Autodesk Inventor part; units mm, degrees
ref_plane "YZ Plane" through (0, 0, 0) normal (1, 0, 0) x (0, 1, 0)
ref_plane "XZ Plane" through (0, 0, 0) normal (0, 1, 0) x (-1, 0, 0)
ref_plane "XY Plane" through (0, 0, 0) normal (0, 0, 1) x (1, 0, 0)
sketch "Sketch1" plane through (0, 0, 0) normal (0, 0, 1) x (1, 0, 0)
  line L0 (2, 0) -> (92, 0)
  line L1 (94, 2) -> (94, 42)
  line L2 (92, 44) -> (2, 44)
  line L3 (0, 42) -> (0, 2)
  line L4 (-1, 47) -> (95, 47)
  line L5 (97, 45) -> (97, -1)
  line L6 (95, -3) -> (-1, -3)
  line L7 (-3, -1) -> (-3, 45)
  arc A0 (2, 44) -> (0, 42) centre (2, 42) ccw
  arc A1 (0, 2) -> (2, 0) centre (2, 2) ccw
  arc A2 (92, 0) -> (94, 2) centre (92, 2) ccw
  arc A3 (94, 42) -> (92, 44) centre (92, 42) ccw
  arc A4 (-3, -1) -> (-1, -3) centre (-1, -1) ccw
  arc A5 (-1, 47) -> (-3, 45) centre (-1, 45) ccw
  arc A6 (97, 45) -> (95, 47) centre (95, 45) ccw
  arc A7 (95, -3) -> (97, -1) centre (95, -1) ccw
  point P0 (0, 0)
  point P1 (94, 44)
  point P2 (94, 0)
  point P3 (0, 44)
  point P4 (97, -3)
  point P5 (97, 47)
  point P6 (-3, -3)
  dimension "d0" = 94
  dimension "d1" = 44
  dimension "d2" = 100
  dimension "d3" = 50
  dimension "d4" = 3
  dimension "d5" = 3
  dimension "d6" = 2
  dimension "d9" = 2
extrude "Extrusion1" add sketch "Sketch1" along normal blind 140
sketch "Sketch2" plane through (0, 0, 140) normal (0, 0, 1) x (1, 0, 0)
  line L0 (-3, 45) -> (-3, -1)
  line L1 (97, -1) -> (97, 45)
  line L2 (-3, 32) -> (97, 32)
  line L3 (97, 32) -> (97, 12)
  line L4 (97, 12) -> (-3, 12)
  line L5 (-3, 12) -> (-3, 32)
  line L6 (-1, -3) -> (95, -3)
  line L7 (95, 47) -> (-1, 47)
  point P0 (0, 0)
  point P1 (-3, 12)
  dimension "d10" = 20
  dimension "d11" = 15
  dimension "d12" = 50
extrude "Extrusion2" cut sketch "Sketch2" against normal blind 2
sketch "Sketch3" plane through (97, -1, 0) normal (1, 0, 0) x (0, 0, -1)
  line L0 (-11, 5.5) -> (-36.5, 5.5)
  line L1 (-37.5, 6.5) -> (-37.5, 15.5)
  line L2 (-36.5, 16.5) -> (-11, 16.5)
  line L3 (-10, 15.5) -> (-10, 6.5)
  line L4 (0, -2) -> (-140, -2)
  line L5 (0, 48) -> (-140, 48)
  line L6 (0, 0) -> (0, 46)
  arc A0 (-11, 5.5) -> (-10, 6.5) centre (-11, 6.5) ccw
  arc A1 (-10, 15.5) -> (-11, 16.5) centre (-11, 15.5) ccw
  arc A2 (-37.5, 6.5) -> (-36.5, 5.5) centre (-36.5, 6.5) ccw
  arc A3 (-36.5, 16.5) -> (-37.5, 15.5) centre (-36.5, 15.5) ccw
  circle A4 centre (-7.09, 11) radius 1.5
  circle A5 centre (-40.41, 11) radius 1.5
  line L7 (-23.75, 5.5) -> (-23.75, 19.7829) construction
  point P0 (0, 1)
  point P1 (-37.5, 16.5)
  point P2 (-37.5, 5.5)
  point P3 (-10, 16.5)
  dimension "d15" = 27.5
  dimension "d16" = 11
  dimension "d17" = 50
  dimension "d18" = 31.5
  dimension "d19" = 10
  dimension "d20" = 1
  dimension "d21" = 3
  dimension "d22" = 3
  dimension "d23" = 16.66
  dimension "d24" = 16.66
extrude "Extrusion3" cut sketch "Sketch3" against normal blind 10 contours L0 A2 L1 A3 L2 A1 L3 A0
hole "Hole1" at (97, 10, 7.09) at (97, 10, 40.41) direction (-1, 0, 0) diameter 3.4 depth 8.8 tip angle 118
chamfer "Chamfer1" distance 0.3 angle 45 2 edges at (97, 10, 8.79) (97, 10, 42.11)
sketch "Sketch5" plane through (-1, -3, 0) normal (0, -1, 0) x (1, 0, 0)
  circle A0 centre (45.75, 3.13) radius 1.5
  circle A1 centre (45.75, 97.75) radius 1.5
  line L0 (98, 0) -> (98, 140)
  line L1 (0, 0) -> (96, 0)
  point P0 (1, 0)
  dimension "d49" = 3
  dimension "d50" = 3
  dimension "d51" = 94.62
  dimension "d52" = 52.25
  dimension "d53" = 3.13
hole "Hole3" at (44.75, -3, 3.13) at (44.75, -3, 97.75) direction (0, 1, 0) diameter 2.6416 depth 10.979 tip angle 118
sketch "Sketch6" plane through (0, 0, 0) normal (0, 0, -1) x (-1, 0, 0)
  circle A0 centre (0.8, -0.8) radius 1
  line L0 (1, -3) -> (-95, -3) construction
  line L1 (-47, -3) -> (-47, -11.0585) construction
  line L2 (3, 45) -> (3, -1) construction
  line L3 (3, 22) -> (17.9543, 22) construction
  circle A1 centre (0.8, 44.8) radius 1
  line L4 (-47, 47) -> (-47, 55.0585) construction
  circle A2 centre (-94.8, -0.8) radius 1
  circle A3 centre (-94.8, 44.8) radius 1
  point P0 (0, 0)
  point P1 (-94, 0)
  point P2 (-97, 45)
  point P3 (-97, -1)
  dimension "d61" = 2
  dimension "d62" = 2.2
  dimension "d63" = 2.2
hole "Hole4" at (-0.8, -0.8, 0) at (-0.8, 44.8, 0) at (94.8, 44.8, 0) at (94.8, -0.8, 0) direction (0, 0, 1) diameter 1.567 depth 6.3 tip angle 118
chamfer "Chamfer2" distance 0.2 angle 45 4 edges at (-0.8, -1.5835, 0) (-0.8, 44.0165, 0) (94.8, 44.0165, 0) (94.8, -1.5835, 0)
equation "\"d24\" = d23"
properties part number "obudowa"
Verification items for the finished model (mm, model axes). A direction names the side the tool comes from. Coordinates: 2 decimals unless noted, no trailing zeros. Order: outer loops, then holes, each group sorted by start corner. A loop starts at its lowest first (then second) coordinate and runs counter-clockwise, first axis right, second up. Notation, with made-up numbers: (80.25, 21) - (129.25, 21) arc R21 cw to (129.25, 60) - close; hole circle Ø5 at (53.25, 73). An arc over 180 degrees is marked (long way). Return JSON: item names as keys, results as strings.
(1) Mould release check, pull along X, two halves, no side actions. Record for faces 1 (the flat face through (97, 22, 69)), 2 (the flat face through (0, 22, 69)), 3 (the flat face through (47, 45, 140)), 4 (the flat face through (46, 0, 69)): pulls with the +X half, pulls with the -X half, needs draft (parallel to the pull), parting line crosses it, or undercut.
Filled sheet:
{"face 1": "pulls with the +X half", "face 2": "undercut", "face 3": "needs draft", "face 4": "undercut"}
(2) Section check D-D, the plane y = 17. Record the cut outline in (x, z).
Filled sheet:
{"outline": "(-3, 0) - (0, 0) - (0, 138) - (-3, 138) - close; (94, 0) - (97, 0) - (97, 138) - (94, 138) - close"}
(3) Thickness scan on line 1 along Z through (x, y) = (95.15, 10); line 2 along X through (y, z) = (17.5, 102); line 3 along Y through (x, z) = (22.5, 71.5). Record the ranges inside material, lowest first.
Filled sheet:
{"line 1": "z = 0 to 5.39, 8.79 to 10, 37.5 to 38.71, 42.11 to 140", "line 2": "x = -3 to 0, 94 to 97", "line 3": "y = -3 to 0, 44 to 47"}
(4) Section check A-A, the plane x = 86. Record the cut outline in (y, z), and give its area (3 significant figures).
Filled sheet:
{"outline": "(-3, 0) - (0, 0) - (0, 140) - (-3, 140) - close; (44, 0) - (47, 0) - (47, 140) - (44, 140) - close", "area": "840 mm^2"}
(5) Access from +Z, -Z, +X, -X, +Y, -Y to the whole of each face (thin tool, end or side, straight path). Record for faces 5 (the cylindrical face through (95.33, 11.66, 7.46)), 6 (the flat face through (48, 44, 69)), 7 (the flat face through (47, -1, 140)), 8 (the flat face through (-2, 22, 138)).
Filled sheet:
{"face 5": "+X", "face 6": "+Z, -Z", "face 7": "+Z, +X, -X, +Y, -Y", "face 8": "+Z, +X, -X"}
(6) Section check C-C, the plane z = 40.41. Record the cut outline in (x, y).
Filled sheet:
{"outline": "(-3, -1) arc R2 ccw to (-1, -3) - (95, -3) arc R2 ccw to (97, -1) - (97, 8) - (96.7, 8.3) - (94, 8.3) - (94, 2) arc R2 cw to (92, 0) - (2, 0) arc R2 cw to (0, 2) - (0, 42) arc R2 cw to (2, 44) - (92, 44) arc R2 cw to (94, 42) - (94, 11.7) - (96.7, 11.7) - (97, 12) - (97, 45) arc R2 ccw to (95, 47) - (-1, 47) arc R2 ccw to (-3, 45) - close"}
(7) Section check B-B, the plane y = 10. Record the cut outline in (x, z).
Filled sheet:
{"outline": "(-3, 0) - (0, 0) - (0, 140) - (-3, 140) - close; (94, 0) - (97, 0) - (97, 5.09) - (96.7, 5.39) - (94, 5.39) - close; (94, 8.79) - (96.7, 8.79) - (97, 9.09) - (97, 10) - (94, 10) - close; (94, 37.5) - (97, 37.5) - (97, 38.41) - (96.7, 38.71) - (94, 38.71) - close; (94, 42.11) - (96.7, 42.11) - (97, 42.41) - (97, 140) - (94, 140) - close"}
(8) Go/stop test with flat-tipped pins: pin 1 (0.6 mm diameter, centred on x = 95.5, z = 139, fed in from -Y); pin 2 (0.9 mm diameter, centred on x = 95.5, y = 21.5, fed in from +Z); pin 3 (0.9 mm diameter, centred on x = -0.8, y = -0.8, fed in from -Z). Record where each tip stops, or that it passes through.
Filled sheet:
{"pin 1": "stops at y = -2.99", "pin 2": "stops at z = 138", "pin 3": "stops at z = 6.5"}
